Read the model definition and answer for the solid it produces. Units are mm, in the model's axes. Face numbers are marked on the shaded views. A direction names the side the tool comes from. Round coordinates to 2 decimals unless told otherwise and drop trailing zeros. Order: outer loops, then holes, each group sorted by start corner. A loop starts at its lowest first (then second) coordinate and runs counter-clockwise, first axis right, second up.
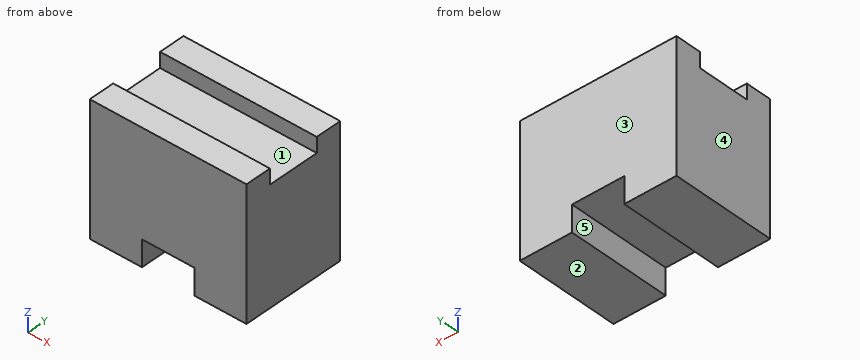
from build123d import *

# Parameters (mm, degrees)
F1_DEPTH = 38.1
F2_W     = 12.7
F2_H     = 6.35
F3_DEPTH = 25.4
F4_DEPTH = 50.8
F5_DEPTH = 25.4


with BuildPart() as f1:
    # F0 (on Right) → F1 (new body)
    with BuildSketch(Plane.YZ):
        Polygon((-12.7, 0), (0, 0), (12.7, 0), (12.7, 31.75), (6.35, 31.75), (6.35, 28.071857), (-6.35, 28.071857), (-6.35, 31.75), (-12.7, 31.75), align=None)
    extrude(amount=F1_DEPTH)

    # F2 (on Front) → F3 (cut)
    with BuildSketch(Plane.XZ):
        with Locations((19.05, 3.175)):
            Rectangle(F2_W, F2_H)
    extrude(amount=-F3_DEPTH, mode=Mode.SUBTRACT)

    # F2 (on Front) → F4 (cut)
    with BuildSketch(Plane.XZ):
        with Locations((19.05, 3.175)):
            Rectangle(F2_W, F2_H)
    extrude(amount=-F4_DEPTH, mode=Mode.SUBTRACT)

    # F2 (on Front) → F5 (cut)
    with BuildSketch(Plane.XZ):
        with Locations((19.05, 3.175)):
            Rectangle(F2_W, F2_H)
    extrude(amount=F5_DEPTH, mode=Mode.SUBTRACT)


solid = f1.part
Q1. A cutting plane is placed at D-D, the plane z = 4. Give the vertices of the cut face in (x, y), plus the area to 3 significant figures.
Outcome:
outline: (0, -12.7) - (12.7, -12.7) - (12.7, 12.7) - (0, 12.7) - close; (25.4, -12.7) - (38.1, -12.7) - (38.1, 12.7) - (25.4, 12.7) - close
area: 645 mm2
Q2. A cutting plane is placed at B-B, the plane y = 9.75. Give the vertices of the cut face in (x, z), plus the area to 3 significant figures.
Outcome:
outline: (0, 0) - (12.7, 0) - (12.7, 6.35) - (25.4, 6.35) - (25.4, 0) - (38.1, 0) - (38.1, 31.75) - (0, 31.75) - close
area: 1,130 mm2
Q3. For the marked faces 4 and 5, determine the directions among +Z, -Z, +X, -X, +Y, -Y from which every point of the face is accessible in a straight line to the end or side of a thin tool.
Outcome:
face 4: +Z, -Z, -X, +Y, -Y
face 5: -Z, +Y, -Y
Q4. A flat-ended cylindrical pin translates along its axis: pin 1 (8 mm diameter, centred on x = 19.5, y = 1, fed in from -Z). Find the tip coordinate at first contact, or state that the pin passes through.
Outcome:
pin 1: stops at z = 6.35
Q5. For a pull along Y with two mould halves and no side action, classify the marked faces 1, 2 and 3 as released by +Y, released by -Y, zero draft, split by the parting line, or undercut.
Outcome:
face 1: undercut
face 2: zero draft
face 3: released by +Y
Q6. A cutting plane is placed at A-A, the plane z = 30. Give the vertices of the cut face in (x, y).
Outcome:
outline: (0, -12.7) - (38.1, -12.7) - (38.1, -6.35) - (0, -6.35) - close; (0, 6.35) - (38.1, 6.35) - (38.1, 12.7) - (0, 12.7) - close
Q7. A cutting plane is placed at C-C, the plane x = 5.5. Give the vertices of the cut face in (y, z).
Outcome:
outline: (-12.7, 0) - (12.7, 0) - (12.7, 31.75) - (6.35, 31.75) - (6.35, 28.07) - (-6.35, 28.07) - (-6.35, 31.75) - (-12.7, 31.75) - close
Q8. Straight lines are drawn through the part: probe 1 along Z at (x, y) = (7, -5.5); probe 2 along Z at (x, y) = (22, 11). For each, find the intervals that lie inside material, in ascending order.
Outcome:
probe 1: z = 0 to 28.07
probe 2: z = 6.35 to 31.75
